Build history of the part. All positions in model axes, mm. Give positions to 0.01 mm unless a question says otherwise; leave off trailing zeros. Write each loop counter-clockwise with the first axis right and the second up, starting at its lowest first coordinate (ties: lowest second). Pieces come first, ordered by that corner, then holes.
from build123d import *

# Parameters (mm, degrees)
SKETCH1_W           = 18.372011154
SKETCH1_H           = 14
SKETCH1_R           = 1
SKETCH1_R_2         = 4
BOSS_EXTRUDE1_DEPTH = 3
CHAMFER1_SIZE       = 3


with BuildPart() as part:
    # Sketch1 → Boss-Extrude1 (new body)
    with BuildSketch(Plane.XY):
        Rectangle(SKETCH1_W, SKETCH1_H)
        with Locations((-6, 0)):
            Circle(SKETCH1_R, mode=Mode.SUBTRACT)
        with Locations((6, 0)):
            Circle(SKETCH1_R, mode=Mode.SUBTRACT)
        Circle(SKETCH1_R_2, mode=Mode.SUBTRACT)
    extrude(amount=BOSS_EXTRUDE1_DEPTH)

    # Chamfer1
    chamfer1_edges = [part.edges().sort_by_distance(p)[0] for p in [
        (9.186005577, -7, 1.5),
        (-9.186005577, -7, 1.5),
        (-9.186005577, 7, 1.5),
        (9.186005577, 7, 1.5),
    ]]
    chamfer(chamfer1_edges, length=CHAMFER1_SIZE)


solid = part.part
1. Saw through at D-D on x = 3.5. Give the cut face in (y, z).
2. Drill centre lines: line 1 along Y through (x, z) = (-6, 1.05); line 2 along X through (y, z) = (-0.5, 1.7); line 3 along Y through (x, z) = (-3.5, 2.1). Where is each one in solid material? Low to high.
3. Saw through at A-A on x = 0. Give the cut face in (y, z), plus the area to 3 significant figures.
4. Mould opens along Y. For faces 1 (the face through (7.707, 5.479, 1.479)), 2 (the face through (7.707, -5.479, 1.479)), 3 (the face through (-0.867, -3.905, 1.479)) say: pulls with the +Y half, pulls with the -Y half, needs draft (parallel to the pull), parting line crosses it, or undercut.
5. Saw through at B-B on y = 0. Give the cut face in (x, z).
6. Saw through at C-C on z = 0.9. Give the cut face in (x, y).
Outcome:
1. outline: (-7, 0) - (-1.94, 0) - (-1.94, 3) - (-7, 3) - close; (1.94, 0) - (7, 0) - (7, 3) - (1.94, 3) - close
2. line 1: y = -7 to -1, 1 to 7
2. line 2: x = -9.19 to -6.87, -5.13 to -3.97, 3.97 to 5.13, 6.87 to 9.19
2. line 3: y = -7 to -1.94, 1.94 to 7
3. outline: (-7, 0) - (-4, 0) - (-4, 3) - (-7, 3) - close; (4, 0) - (7, 0) - (7, 3) - (4, 3) - close
3. area: 18.0 mm2
4. face 1: pulls with the +Y half
4. face 2: pulls with the -Y half
4. face 3: undercut
5. outline: (-9.19, 0) - (-7, 0) - (-7, 3) - (-9.19, 3) - close; (-5, 0) - (-4, 0) - (-4, 3) - (-5, 3) - close; (4, 0) - (5, 0) - (5, 3) - (4, 3) - close; (7, 0) - (9.19, 0) - (9.19, 3) - (7, 3) - close
6. outline: (-9.19, -4) - (-6.19, -7) - (6.19, -7) - (9.19, -4) - (9.19, 4) - (6.19, 7) - (-6.19, 7) - (-9.19, 4) - close; hole circle Ø2 at (-6, 0); hole circle Ø8 at (0, 0); hole circle Ø2 at (6, 0)
